Source: CAD feature listing. Evaluate the final solid. Frame: model axes, mm. Give positions to 0.01 mm unless a question says otherwise; leave off trailing zeros. Write each loop counter-clockwise with the first axis right and the second up, starting at its lowest first coordinate (ties: lowest second). Pieces come first, ordered by that corner, then holes. Notation, with made-up numbers: M 19.25,28.5 L 68.25,28.5 A16 cw 68.25,41.5 Z; hole C 23.25,54.5 d2. An arc over 180 degrees is marked long. Return JSON: item names as keys, results as strings.
```python
from build123d import *

# Parameters (mm, degrees)
F1_W      = 8.89
F1_H      = 3.175
F3_R      = 2.38125
F4_DEPTH  = 3.176
F7_DEPTH  = 3.176
F8_R      = 5.08
F9_R      = 27.6252152017
F10_DEPTH = 17.4535782288
F11_R     = 14.5350936127
F12_DEPTH = 3.175


# Not quite as in the source:
# - a fillet or chamfer that OpenCascade refuses, or shapes differently, is made with other operations: its cross-section is extruded or revolved along the edge and cut away or added


with BuildPart() as f2:
    # F1 (on Front) → F2 (revolve)
    with BuildSketch(Plane.XZ):
        with BuildLine():
            ThreePointArc((13.208, -11.9177163316), (13.0652297207, -14.7887805254), (12.3057501177, -17.5612494052))
            Line((12.3057501177, -17.5612494052), (16.383, -17.5612494052))
            Line((16.383, -17.5612494052), (16.383, 0))
            Line((16.383, 0), (16.383, 3.175))
            Line((16.383, 3.175), (13.208, 3.175))
            Line((13.208, 3.175), (13.208, -11.9177163316))
        make_face()
        with Locations((20.828, 1.5875)):
            Rectangle(F1_W, F1_H)
    revolve(axis=Axis((0, 0, -9.4681101426), (0, 0, 1)))

    # F3 (on face) → F4 (cut, through all)
    with BuildSketch(Plane(origin=(0, 0, 0), x_dir=(1, 0, 0), z_dir=(0, 0, -1))):
        with BuildLine():
            ThreePointArc((0, 17.93875), (1.6837980227, 18.6362019773), (2.38125, 20.32))
            ThreePointArc((2.38125, 20.32), (-1.6837980227, 22.0037980227), (0, 17.93875))
        make_face()
        with Locations((-17.5976362049, -10.16)):
            Circle(F3_R)
        with Locations((17.5976362049, -10.16)):
            Circle(F3_R)
    extrude(amount=-F4_DEPTH, mode=Mode.SUBTRACT)

    # F5: fillet of radius 5.08 on 1 edges, made by hand

    # F5_s1 → F5_t2 (revolve, cut)
    with BuildSketch(Plane.XZ):
        with BuildLine():
            ThreePointArc((11.303, -17.5612494052), (14.8951024484, -16.0733518536), (16.383, -12.4812494052))
            Line((16.383, -12.4812494052), (16.383, -17.5612494052))
            Line((16.383, -17.5612494052), (11.303, -17.5612494052))
        make_face()
    revolve(axis=Axis((0, 0, -17.5612494052), (0, 0, 1)), mode=Mode.SUBTRACT)

    # F6 (on face) → F7 (cut, through all)
    with BuildSketch(Plane(origin=(0, 0, 0), x_dir=(1, 0, 0), z_dir=(0, 0, -1))):
        with BuildLine():
            ThreePointArc((-4.952964542, 20.3387415379), (-3.495667473, 23.8289197652), (0, 25.273))
            ThreePointArc((0, 25.273), (-21.8870601005, 12.6364998776), (-21.8870598885, -12.6365002448))
            ThreePointArc((-21.8870598885, -12.6365002448), (-22.3842836342, -8.8871231844), (-20.0903491238, -5.8799776515))
            ThreePointArc((-20.0903491238, -5.8799776515), (-18.1286292594, 10.4665689829), (-4.952964542, 20.3387415379))
        make_face()
        with BuildLine():
            ThreePointArc((0, 25.273), (3.495667473, 23.8289197652), (4.952964542, 20.3387415379))
            ThreePointArc((4.952964542, 20.3387415379), (18.1286292594, 10.4665689829), (20.0903491238, -5.8799776515))
            ThreePointArc((20.0903491238, -5.8799776515), (21.8917377458, -7.6916197707), (22.5506362049, -10.16))
            ThreePointArc((22.5506362049, -10.16), (22.3818668231, -11.4419307281), (21.8870600322, -12.6364999959))
            ThreePointArc((21.8870600322, -12.6364999959), (24.4118434084, -6.5411337246), (25.273, 0))
            ThreePointArc((25.273, 0), (17.8707096809, 17.8707096809), (0, 25.273))
        make_face()
        with BuildLine():
            ThreePointArc((-15.1373845818, -14.4587638864), (-18.8886159884, -14.9417967542), (-21.8870598885, -12.6365002448))
            ThreePointArc((-21.8870598885, -12.6365002448), (1.437e-07, -25.273), (21.8870600322, -12.6364999959))
            ThreePointArc((21.8870600322, -12.6364999959), (18.8886161272, -14.9417967167), (15.1373845818, -14.4587638864))
            ThreePointArc((15.1373845818, -14.4587638864), (0, -20.9331379659), (-15.1373845818, -14.4587638864))
        make_face()
    extrude(amount=-F7_DEPTH, mode=Mode.SUBTRACT)

    # F8
    f8_edges = [f2.edges().sort_by_distance(p)[0] for p in [
        (-15.137385, 14.458764, 1.5875),
        (15.137385, 14.458764, 1.5875),
        (20.090349, 5.879978, 1.5875),
        (4.952965, -20.338742, 1.5875),
        (-4.952965, -20.338742, 1.5875),
        (-20.090349, 5.879978, 1.5875),
    ]]
    fillet(f8_edges, radius=F8_R)

    # F9 (on Top) → F10 (cut, through all)
    with BuildSketch(Plane.XY):
        Circle(F9_R)
    extrude(amount=-F10_DEPTH, mode=Mode.SUBTRACT)

    # F11 (on face) → F12 (join)
    with BuildSketch(Plane(origin=(0, 0, 0), x_dir=(1, 0, 0), z_dir=(0, 0, -1))):
        Circle(F11_R)
    extrude(amount=-F12_DEPTH)


solid = f2.part
```
1) Cut plane A-A, the plane x = -1. Return the cut outline in (y, z) (3 decimals).
Numbers:
{"outline": "M -25.171,0 L -22.481,0 L -22.481,3.175 L -25.171,3.175 Z; M -18.159,0 L 20.909,0 L 20.909,3.175 L -18.159,3.175 Z"}
2) Line query: line 1 (X direction, y = 10.16, z = 1.2); line 2 (X direction, y = -18.5, z = 1.45); line 3 (X direction, y = 17, z = 0.25). Output: solid intervals per line, ascending. Write a range as [from, to].
Numbers:
{"line 1": "x = [-22.55, -19.98], [-15.22, 15.22], [19.98, 22.55]", "line 2": "x = [-9.8, -1.54], [1.54, 9.8]", "line 3": "x = [-12.21, 12.21]"}
3) Cut plane B-B, the plane y = 11. Return the cut outline in (x, z) (3 decimals).
Numbers:
{"outline": "M -22.479,0 L -19.826,0 L -19.826,3.175 L -22.479,3.175 Z; M -15.369,0 L 15.369,0 L 15.369,3.175 L -15.369,3.175 Z; M 19.826,0 L 22.479,0 L 22.479,3.175 L 19.826,3.175 Z"}
4) Cut plane C-C, the plane z = 2.1. Give the number of separate pieces and of enclosed holes in the cut face, then the cut area to 3 significant figures.
Numbers:
{"separate pieces": "1", "enclosed holes": "3", "area": "1,430 mm²"}
5) Draft query along Y for faces 1 (the face through (0, -2, 3.175)), 2 (the face through (-0.31, -22.68, 1.57)), 3 (the face through (-15.326, 9.445, 1.565)), 4 (the face through (0.201, 20.932, 1.565)). Return one class per face: released by +Y, released by -Y, zero draft, split by the parting line, or undercut.
Numbers:
{"face 1": "zero draft", "face 2": "undercut", "face 3": "undercut", "face 4": "released by +Y"}
6) Cut plane D-D, the plane y = -6.5. Return the cut outline in (x, z) (3 decimals), then the cut area to 3 significant figures.
Numbers:
{"outline": "M -19.898,0 L 19.898,0 L 19.898,3.175 L -19.898,3.175 Z", "area": "126 mm²"}
7) Contact query for flat-ended pins moving along their axis: pin 1 Ø1.5 at (x, z) = (-3, 1) entering from -Y; pin 2 Ø1 at (x, z) = (-16.5, 1.5) entering from +Y; pin 3 Ø7.5 at (x, y) = (0, -20.32) entering from -Z; pin 4 Ø1.5 at (x, z) = (-6, 2) entering from +Y. Output: stop coordinate, or through.
Numbers:
{"pin 1": "stops at y = -24.73", "pin 2": "stops at y = 15.08", "pin 3": "stops at z = 0", "pin 4": "stops at y = 20.26"}
